Answer from the drawing. Dimensions are ordinates in mm from the lowest x, y and z of the part. A direction names the side the tool comes from. Give positions to 0.01 mm unless a question says otherwise; leave off trailing zeros. Write each loop counter-clockwise with the first axis right and the second up, starting at its lowest first coordinate (ties: lowest second). Pieces come first, ordered by that corner, then holes. Notation, with made-up numbers: (-14, -1.5) -> (27, -1.5) arc R18 ccw to (27, 23.5) -> close; hole circle Ø5 at (48.5, 42.25). An arc over 180 degrees is marked (long way). Use a Markdown table: item, result. Add a question column.
Q1. Consider line 1 (X direction, y = 9, z = 53); line 2 (Z direction, x = 73, y = 37.5); line 3 (Y direction, x = 11.5, z = 28). Determine where each line is inside the solid, lowest interval first.
Q2. Each of these flat-tipped pins is pushed along its axis until it touches: pin 1 Ø7 at (x, z) = (34.5, 52.5) entering from -Y; pin 2 Ø3 at (y, z) = (36.5, 40) entering from -X. Where does it stop, or does it pass through?
Q3. Section C-C, the plane z = 4 is taken. Give the vertices of the cut face in (x, y).
Q4. Section D-D, the plane z = 43.5 is taken. Give the vertices of the cut face in (x, y).
Q5. Section A-A, the plane y = 29 is taken. Give the vertices of the cut face in (x, z).
Q6. For the marked faces 4, 5, 6, 7 and 8, determine the directions among +Z, -Z, +X, -X, +Y, -Y from which every point of the face is accessible in a straight line to the end or side of a thin tool.
Q7. For a pull along Z with two mould halves and no side action, classify the marked faces 1, 2 and 3 as pulls with the +Z half, pulls with the -Z half, needs draft (parallel to the pull), parting line crosses it, or undercut.
Q8. Section B-B, the plane x = 51 is taken. Give the vertices of the cut face in (y, z).
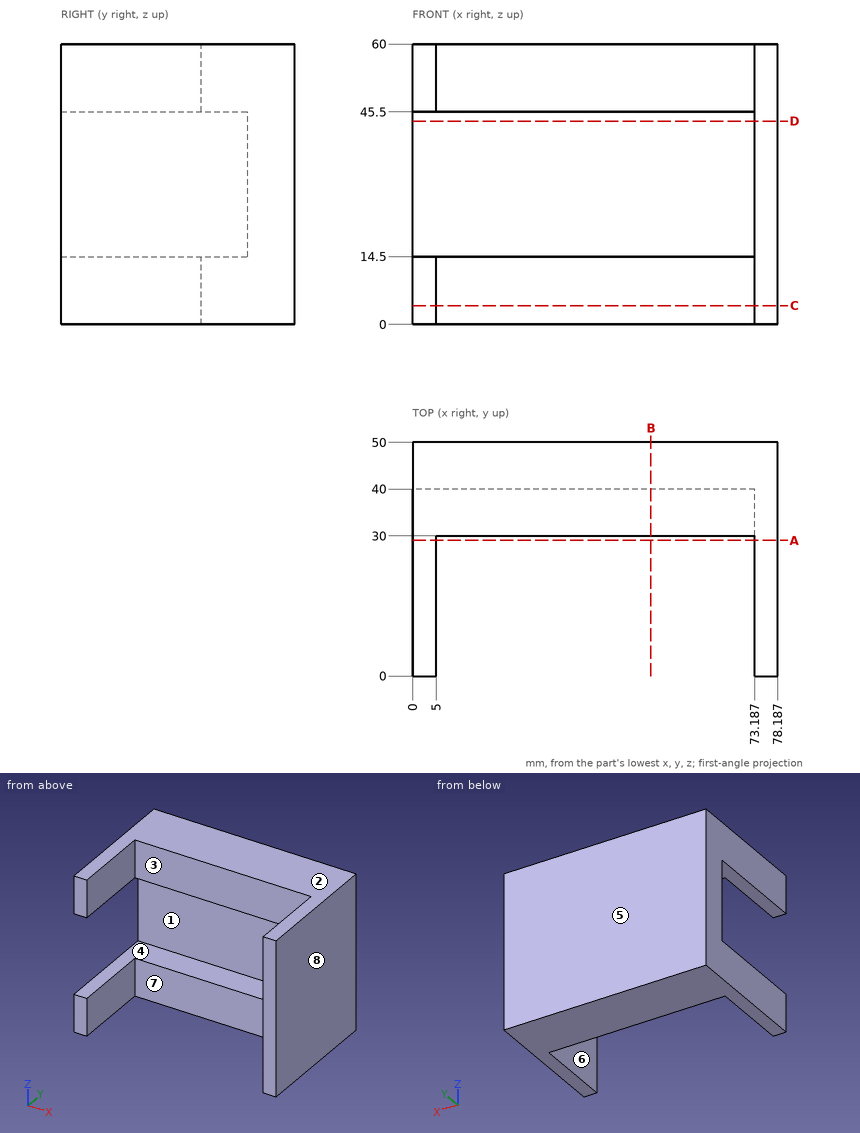
Result set:
| question | item | result |
|---|---|---|
| 1 | line 1 | x = 0 to 5, 73.19 to 78.19 |
| 1 | line 2 | z = 0 to 14.5, 45.5 to 60 |
| 1 | line 3 | y = 40 to 50 |
| 2 | pin 1 | stops at y = 30 |
| 2 | pin 2 | stops at x = 73.19 |
| 3 | outline | (0, 0) -> (5, 0) -> (5, 30) -> (73.19, 30) -> (73.19, 0) -> (78.19, 0) -> (78.19, 50) -> (0, 50) -> close |
| 4 | outline | (0, 40) -> (73.19, 40) -> (73.19, 0) -> (78.19, 0) -> (78.19, 50) -> (0, 50) -> close |
| 5 | outline | (0, 0) -> (5, 0) -> (5, 14.5) -> (0, 14.5) -> close; (0, 45.5) -> (5, 45.5) -> (5, 60) -> (0, 60) -> close; (73.19, 0) -> (78.19, 0) -> (78.19, 60) -> (73.19, 60) -> close |
| 6 | face 4 | -X, -Y |
| 6 | face 5 | +Z, -Z, +X, -X, +Y |
| 6 | face 6 | -Y |
| 6 | face 7 | +Z, -Z, -Y |
| 6 | face 8 | +Z, -Z, +X, +Y, -Y |
| 7 | face 1 | undercut |
| 7 | face 2 | pulls with the +Z half |
| 7 | face 3 | needs draft |
| 8 | outline | (30, 0) -> (50, 0) -> (50, 60) -> (30, 60) -> (30, 45.5) -> (40, 45.5) -> (40, 14.5) -> (30, 14.5) -> close |
